Input: part model. Units: mm. Frame: model coordinates. Give positions to 0.01 mm unless a question says otherwise; leave off trailing zeros. Loops run counter-clockwise (first coordinate to the right, second up) from the corner with the lowest first, then second, coordinate; pieces in that order, holes last. Notation, with made-up numbers: M 39.25,0 L 53.25,0 A20 ccw 53.25,16 Z; hole C 34.25,3.5 d7. An arc over 180 degrees is marked long. Answer as a JSON object with one key per item and string values. Group by question number.
1) Section query A-A on y = 0. Return loops of the section in (x, z).
2) Section query C-C on x = 15. Return loops of the section in (y, z).
3) Section query D-D on y = 17.5. Return loops of the section in (x, z), plus the area to 3 significant figures.
4) First-contact query: P1, Ø0.6, axis at x = 26.5, z = 1.5, coming from the +Y side; P2, Ø0.8, axis at y = 2, z = 0.5, coming from the -X side; P3, Ø0.8, axis at y = 2, z = 1, coming from the +X side. Flat tips, straight axial feed; report the tip coordinate or a pass-through.
5) Section query B-B on x = 0. Return loops of the section in (y, z), plus the area to 3 significant figures.
6) Ray query, L1, parallel to Y at x = 0, z = 1; L2, parallel to Y at x = -36.5, z = 0.9; L3, parallel to X at y = -19, z = 1.4. Return the intervals inside material, ascending.
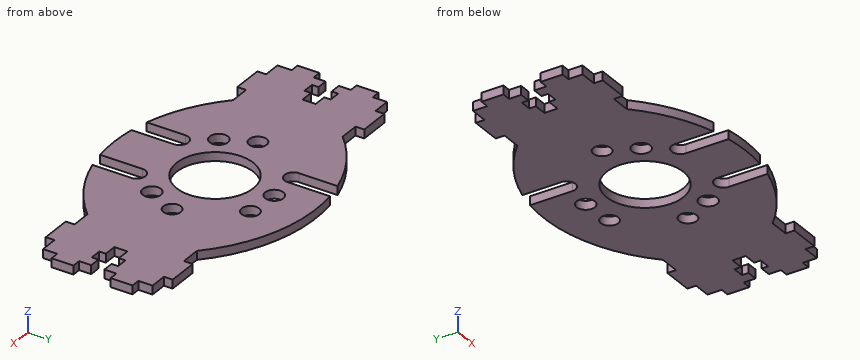
from build123d import *

# Parameters (mm, degrees)
SKETCH_1_R      = 2
SKETCH_1_R_2    = 2.08
SKETCH_1_R_3    = 8.75
EXTRUDE_2_DEPTH = 2


with BuildPart() as part:
    # 草图1 → 凸台-拉伸2 (new body)
    with BuildSketch(Plane.XY):
        with BuildLine():
            Line((-41, 4.25), (-43, 4.25))
            Line((-43, 4.25), (-43, 9.25))
            Line((-43, 9.25), (-41, 9.25))
            Line((-41, 9.25), (-41, 12.5))
            Line((-41, 12.5), (-37, 12.5))
            Line((-37, 12.5), (-37, 14.5))
            Line((-37, 14.5), (-30, 14.5))
            Line((-30, 14.5), (-30, 12.5))
            Line((-30, 12.5), (-25.488968202, 12.5))
            ThreePointArc((-25.488968202, 12.5), (-18.099802413, 18.184292016), (-9.5, 21.783506545))
            Line((-9.5, 21.783506545), (-9.5, 12.990381057))
            ThreePointArc((-9.5, 12.990381057), (-7.5, 10.990381057), (-5.5, 12.990381057))
            Line((-5.5, 12.990381057), (-5.5, 22.635812499))
            ThreePointArc((-5.5, 22.635812499), (11.205953159, 21.271820081), (25.488968202, 12.5))
            Line((25.488968202, 12.5), (30, 12.5))
            Line((30, 12.5), (30, 14.5))
            Line((30, 14.5), (37, 14.5))
            Line((37, 14.5), (37, 12.5))
            Line((37, 12.5), (41, 12.5))
            Line((41, 12.5), (41, 9.25))
            Line((41, 9.25), (43, 9.25))
            Line((43, 9.25), (43, 4.25))
            Line((43, 4.25), (41, 4.25))
            Line((41, 4.25), (41, 1.5))
            Line((41, 1.5), (38.5, 1.5))
            Line((38.5, 1.5), (38.5, 3))
            Line((38.5, 3), (35.9, 3))
            Line((35.9, 3), (35.9, 1.5))
            Line((35.9, 1.5), (32.9, 1.5))
            Line((32.9, 1.5), (32.9, -1.5))
            Line((32.9, -1.5), (35.9, -1.5))
            Line((35.9, -1.5), (35.9, -3))
            Line((35.9, -3), (38.5, -3))
            Line((38.5, -3), (38.5, -1.5))
            Line((38.5, -1.5), (41, -1.5))
            Line((41, -1.5), (41, -4.25))
            Line((41, -4.25), (43, -4.25))
            Line((43, -4.25), (43, -9.25))
            Line((43, -9.25), (41, -9.25))
            Line((41, -9.25), (41, -12.5))
            Line((41, -12.5), (37, -12.5))
            Line((37, -12.5), (37, -14.5))
            Line((37, -14.5), (30, -14.5))
            Line((30, -14.5), (30, -12.5))
            Line((30, -12.5), (25.488968202, -12.5))
            ThreePointArc((25.488968202, -12.5), (18.099802413, -18.184292016), (9.5, -21.783506545))
            Line((9.5, -21.783506545), (9.5, -12.990381057))
            ThreePointArc((9.5, -12.990381057), (7.5, -10.990381057), (5.5, -12.990381057))
            Line((5.5, -12.990381057), (5.5, -22.635812499))
            ThreePointArc((5.5, -22.635812499), (0, -23.05787632), (-5.5, -22.635812499))
            Line((-5.5, -22.635812499), (-5.5, -12.990381057))
            ThreePointArc((-5.5, -12.990381057), (-7.5, -10.990381057), (-9.5, -12.990381057))
            Line((-9.5, -12.990381057), (-9.5, -21.783506545))
            ThreePointArc((-9.5, -21.783506545), (-18.099802413, -18.184292016), (-25.488968202, -12.5))
            Line((-25.488968202, -12.5), (-30, -12.5))
            Line((-30, -12.5), (-30, -14.5))
            Line((-30, -14.5), (-37, -14.5))
            Line((-37, -14.5), (-37, -12.5))
            Line((-37, -12.5), (-41, -12.5))
            Line((-41, -12.5), (-41, -9.25))
            Line((-41, -9.25), (-43, -9.25))
            Line((-43, -9.25), (-43, -4.25))
            Line((-43, -4.25), (-41, -4.25))
            Line((-41, -4.25), (-41, -1.5))
            Line((-41, -1.5), (-38.5, -1.5))
            Line((-38.5, -1.5), (-38.5, -3))
            Line((-38.5, -3), (-35.9, -3))
            Line((-35.9, -3), (-35.9, -1.5))
            Line((-35.9, -1.5), (-32.9, -1.5))
            Line((-32.9, -1.5), (-32.9, 1.5))
            Line((-32.9, 1.5), (-35.9, 1.5))
            Line((-35.9, 1.5), (-35.9, 3))
            Line((-35.9, 3), (-38.5, 3))
            Line((-38.5, 3), (-38.5, 1.5))
            Line((-38.5, 1.5), (-41, 1.5))
            Line((-41, 1.5), (-41, 4.25))
        make_face()
        with Locations((-15, 0)):
            Circle(SKETCH_1_R, mode=Mode.SUBTRACT)
        with Locations((7.5, 12.990381057)):
            Circle(SKETCH_1_R, mode=Mode.SUBTRACT)
        with Locations((15, 0)):
            Circle(SKETCH_1_R, mode=Mode.SUBTRACT)
        with Locations((0, 13.53)):
            Circle(SKETCH_1_R_2, mode=Mode.SUBTRACT)
        with Locations((11.717323713, -6.765)):
            Circle(SKETCH_1_R_2, mode=Mode.SUBTRACT)
        with Locations((-11.717323713, -6.765)):
            Circle(SKETCH_1_R_2, mode=Mode.SUBTRACT)
        Circle(SKETCH_1_R_3, mode=Mode.SUBTRACT)
    extrude(amount=EXTRUDE_2_DEPTH)


solid = part.part
Output:
{
 "1": {"outline": "M -32.9,0 L -17,0 L -17,2 L -32.9,2 Z; M -13,0 L -8.75,0 L -8.75,2 L -13,2 Z; M 8.75,0 L 13,0 L 13,2 L 8.75,2 Z; M 17,0 L 32.9,0 L 32.9,2 L 17,2 Z"},
 "2": {"outline": "M -19.79,0 L -2,0 L -2,2 L -19.79,2 Z; M 2,0 L 19.79,0 L 19.79,2 L 2,2 Z"},
 "3": {"outline": "M -19.23,0 L -9.5,0 L -9.5,2 L -19.23,2 Z; M -5.5,0 L 19.23,0 L 19.23,2 L -5.5,2 Z", "area": "68.9 mm^2"},
 "4": {"P1": "stops at y = 12.5", "P2": "stops at x = -41", "P3": "stops at x = 41"},
 "5": {"outline": "M -23.06,0 L -8.75,0 L -8.75,2 L -23.06,2 Z; M 8.75,0 L 11.45,0 L 11.45,2 L 8.75,2 Z; M 15.61,0 L 23.06,0 L 23.06,2 L 15.61,2 Z", "area": "48.9 mm^2"},
 "6": {"L1": "y = -23.06 to -8.75, 8.75 to 11.45, 15.61 to 23.06", "L2": "y = -14.5 to -3, 3 to 14.5", "L3": "x = -16.62 to -9.5, -5.5 to 5.5, 9.5 to 16.62"}
}
